Model file for the job. Use its own axes, mm. Round coordinates to 2 decimals unless told otherwise and drop trailing zeros. Loops run counter-clockwise (first coordinate to the right, second up) from the corner with the lowest first, then second, coordinate; pieces in that order, holes last. Notation, with made-up numbers: (-31.5, -20) - (-16.5, -20) arc R11 ccw to (-16.5, -5) - close; hole circle Ø4 at (-24.75, 54.5). An arc over 180 degrees is marked (long way). Answer as a JSON object with one key per item and string values.
from build123d import *

# Parameters (mm, degrees)
SKETCH2_R           = 4
BOSS_EXTRUDE1_DEPTH = 5
SKETCH3_R           = 2
CUT_EXTRUDE1_DEPTH  = 5


with BuildPart() as part:
    # Sketch2 → Boss-Extrude1 (new body)
    with BuildSketch(Plane.XY):
        Polygon((75, 300), (75, -200), (135, -200), (135, -250), (75, -250), (75, -300), (-75, -300), (-75, -250), (-135, -250), (-135, -200), (-75, -200), (-75, 300), align=None)
        with Locations((-105, -225)):
            Circle(SKETCH2_R, mode=Mode.SUBTRACT)
        with Locations((105, -225)):
            Circle(SKETCH2_R, mode=Mode.SUBTRACT)
    extrude(amount=BOSS_EXTRUDE1_DEPTH)

    # Sketch3 → Cut-Extrude1 (cut)
    with BuildSketch(Plane.XY.offset(5)):
        with Locations((-52.5, 280)):
            Circle(SKETCH3_R)
        with Locations((-52.5, 220)):
            Circle(SKETCH3_R)
        with Locations((-52.5, 160)):
            Circle(SKETCH3_R)
        with Locations((-52.5, 100)):
            Circle(SKETCH3_R)
        with Locations((-52.5, 40)):
            Circle(SKETCH3_R)
        with Locations((-52.5, -20)):
            Circle(SKETCH3_R)
        with Locations((-52.5, -80)):
            Circle(SKETCH3_R)
        with Locations((-52.5, -140)):
            Circle(SKETCH3_R)
        with Locations((-52.5, -200)):
            Circle(SKETCH3_R)
        with Locations((-52.5, -260)):
            Circle(SKETCH3_R)
        with Locations((52.5, -260)):
            Circle(SKETCH3_R)
        with Locations((52.5, -200)):
            Circle(SKETCH3_R)
        with Locations((52.5, -140)):
            Circle(SKETCH3_R)
        with Locations((52.5, -80)):
            Circle(SKETCH3_R)
        with Locations((52.5, -20)):
            Circle(SKETCH3_R)
        with Locations((52.5, 40)):
            Circle(SKETCH3_R)
        with Locations((52.5, 100)):
            Circle(SKETCH3_R)
        with Locations((52.5, 160)):
            Circle(SKETCH3_R)
        with Locations((52.5, 220)):
            Circle(SKETCH3_R)
        with Locations((52.5, 280)):
            Circle(SKETCH3_R)
    extrude(amount=-CUT_EXTRUDE1_DEPTH, mode=Mode.SUBTRACT)


solid = part.part
1) Slice it at B-B on y = -189. List the corners of the cut face in (x, z).
Values follow:
{"outline": "(-75, 0) - (75, 0) - (75, 5) - (-75, 5) - close"}
2) Drop flat-ended pins along their axis: P1, Ø3.5, axis at x = 52.5, y = -20, coming from the -Z side; P2, Ø2.5, axis at x = -91, z = 1.5, coming from the -Y side; P3, Ø1.5, axis at y = -274, z = 3.5, coming from the +X side. Give the stop position or say it passes through.
Values follow:
{"P1": "through", "P2": "y = -250", "P3": "x = 75"}
3) Slice it at A-A on z = 2.85. Count the separate pieces of the cut face and the enclosed holes in it, then the cut area to 3 significant figures.
Values follow:
{"separate pieces": "1", "enclosed holes": "22", "area": "95,600 mm²"}
4) Probe probe 1 along X at (y, z) = (-260, 3.7); probe 2 along X at (y, z) = (219.5, 3.8); probe 3 along Y at (x, z) = (111.5, 1.5). List the from-to ranges inside material, lowest first.
Values follow:
{"probe 1": "-75 to -54.5, -50.5 to 50.5, 54.5 to 75", "probe 2": "-75 to -54.44, -50.56 to 50.56, 54.44 to 75", "probe 3": "-250 to -200"}
